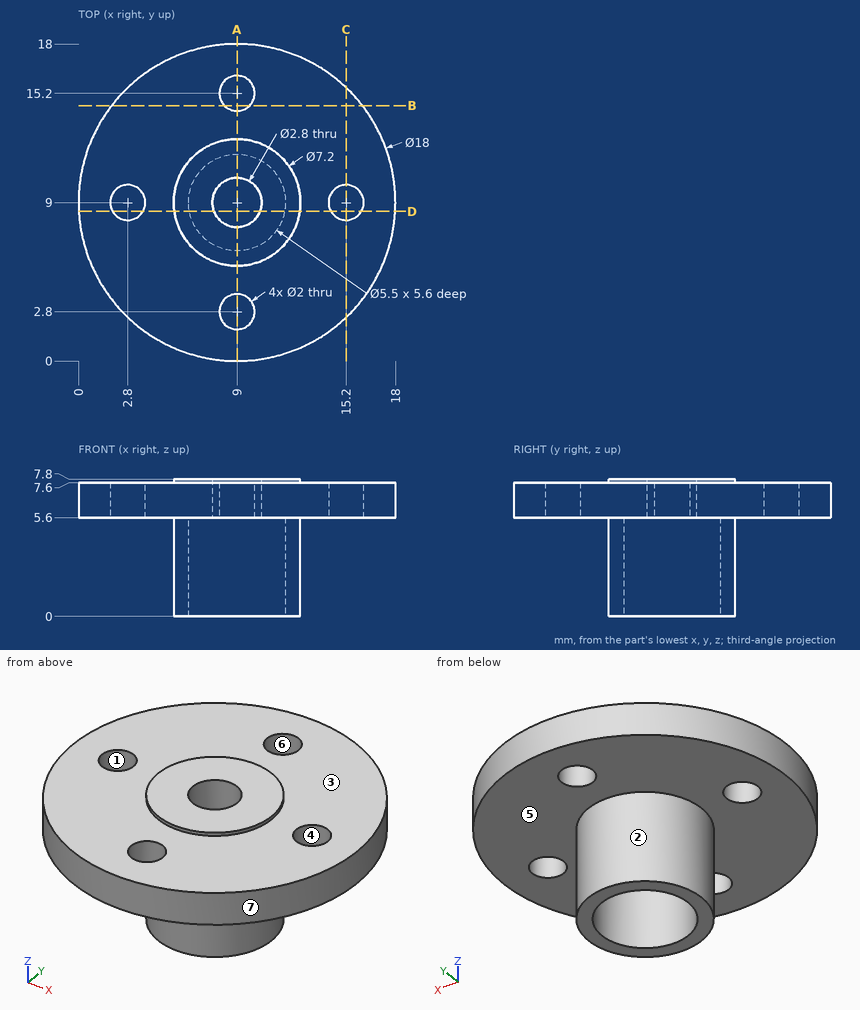
Input: dimensioned drawing with shaded views. Units: mm. Origin: part minimum x, y, z. A direction names the side the tool comes from. Round coordinates to 2 decimals unless told otherwise and drop trailing zeros. Order: outer loops, then holes, each group sorted by start corner. A loop starts at its lowest first (then second) coordinate and runs counter-clockwise, first axis right, second up.
1. Cut plane B-B, the plane y = 14.5. Output: boundary loops of the cut face in (x, z), then the cut area to 3 significant figures.
The answers:
outline: (1.88, 5.6) - (8.29, 5.6) - (8.29, 7.6) - (1.88, 7.6) - close; (9.71, 5.6) - (16.12, 5.6) - (16.12, 7.6) - (9.71, 7.6) - close
area: 25.6 mm2
2. Set-up query: the marked faces 1, 2 and 3. Return all of +Z, -Z, +X, -X, +Y, -Y with unobstructed straight access to the full face (end or side cutting, diameter ignored); none if empty.
The answers:
face 1: +Z, -Z
face 2: -Z
face 3: +Z
3. Cut plane D-D, the plane y = 8.5. Output: boundary loops of the cut face in (x, z).
The answers:
outline: (0.01, 5.6) - (1.93, 5.6) - (1.93, 7.6) - (0.01, 7.6) - close; (3.67, 5.6) - (5.43, 5.6) - (5.43, 0) - (6.3, 0) - (6.3, 5.6) - (7.69, 5.6) - (7.69, 7.8) - (5.43, 7.8) - (5.43, 7.6) - (3.67, 7.6) - close; (10.31, 5.6) - (11.7, 5.6) - (11.7, 0) - (12.57, 0) - (12.57, 5.6) - (14.33, 5.6) - (14.33, 7.6) - (12.57, 7.6) - (12.57, 7.8) - (10.31, 7.8) - close; (16.07, 5.6) - (17.99, 5.6) - (17.99, 7.6) - (16.07, 7.6) - close
4. Pin query (flat end, axial travel): P1, Ø3, axis at x = 9, y = 15.2, coming from the -Z side; P2, Ø1.5, axis at y = 2.5, z = 6, coming from the +X side; P3, Ø2.5, axis at x = 2.8, y = 9, coming from the +Z side. Return the tip coordinate at first contact, or that it passes through.
The answers:
P1: stops at z = 5.6
P2: stops at x = 15.92
P3: stops at z = 7.6
5. Mould query, pull axis Y, two halves, no side actions, for the marked faces 4, 5, 6 and 7. Classes: released by +Y, released by -Y, zero draft, split by the parting line, or undercut.
The answers:
face 4: undercut
face 5: zero draft
face 6: undercut
face 7: split by the parting line
6. Cut plane C-C, the plane x = 15.2. Output: boundary loops of the cut face in (y, z), then the cut area to 3 significant figures.
The answers:
outline: (2.48, 5.6) - (8, 5.6) - (8, 7.6) - (2.48, 7.6) - close; (10, 5.6) - (15.52, 5.6) - (15.52, 7.6) - (10, 7.6) - close
area: 22.1 mm2
7. Material intervals for line 1 (Y direction, x = 9, z = 7.1); line 2 (Y direction, x = 9, z = 4.4); line 3 (Z direction, x = 12.5, y = 11.75), sorted ascending.
The answers:
line 1: y = 0 to 1.8, 3.8 to 7.6, 10.4 to 14.2, 16.2 to 18
line 2: y = 5.4 to 6.25, 11.75 to 12.6
line 3: z = 5.6 to 7.6
8. Cut plane A-A, the plane x = 9. Output: boundary loops of the cut face in (y, z).
The answers:
outline: (0, 5.6) - (1.8, 5.6) - (1.8, 7.6) - (0, 7.6) - close; (3.8, 5.6) - (5.4, 5.6) - (5.4, 0) - (6.25, 0) - (6.25, 5.6) - (7.6, 5.6) - (7.6, 7.8) - (5.4, 7.8) - (5.4, 7.6) - (3.8, 7.6) - close; (10.4, 5.6) - (11.75, 5.6) - (11.75, 0) - (12.6, 0) - (12.6, 5.6) - (14.2, 5.6) - (14.2, 7.6) - (12.6, 7.6) - (12.6, 7.8) - (10.4, 7.8) - close; (16.2, 5.6) - (18, 5.6) - (18, 7.6) - (16.2, 7.6) - close
